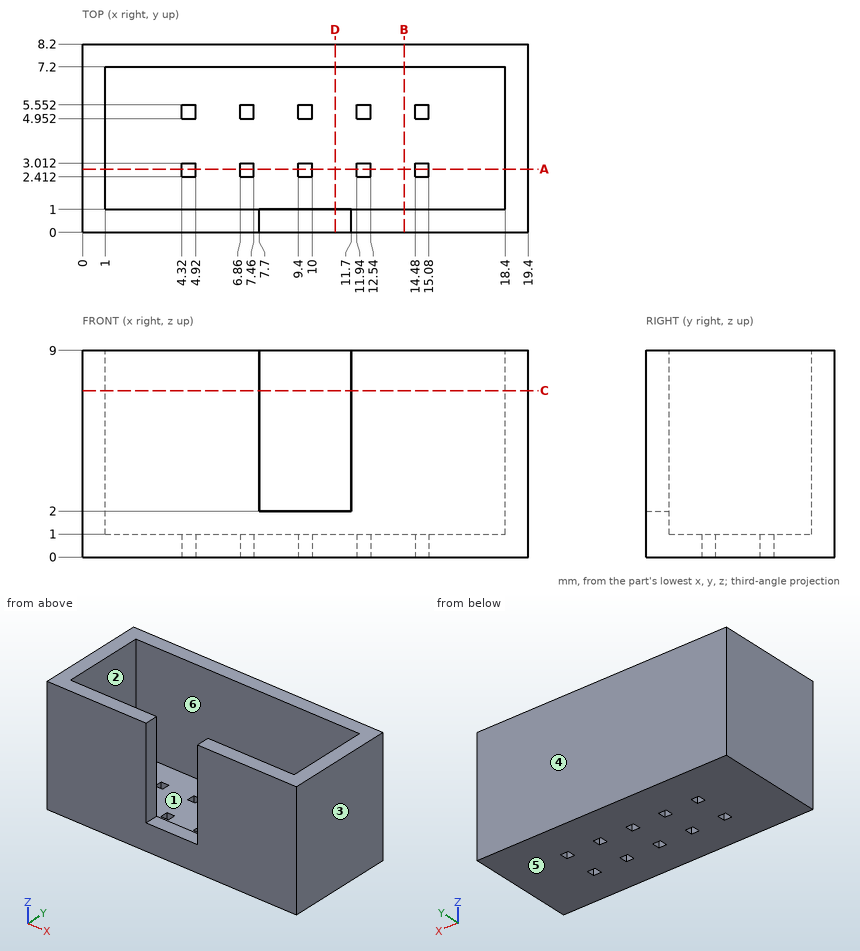
Could you check a few things on this drawing? It's one solid part, dimensions in mm from its lowest x, y, z. A direction names the side the tool comes from. Give positions to 0.01 mm unless a question says otherwise; leave off trailing zeros. Order: outer loops, then holes, each group sorted by start corner. A loop starts at its lowest first (then second) coordinate and runs counter-clockwise, first axis right, second up. Notation, with made-up numbers: (32, 77.5) - (78, 77.5) arc R27 ccw to (78, 108.5) - close; hole circle Ø2 at (-13, 27). An arc over 180 degrees is marked (long way). Answer as a JSON object with one key per item and string values. Group by question number.
Item 1: If we section it at A-A on y = 2.75: Please give me the cut outline in (x, z).
Item 2: Which directions (+Z, -Z, +X, -X, +Y, -Y) give clear straight access to the entire face, cutting with the end or side of a thin tool? Please do the marked faces 5 and 6.
Item 3: If we section it at D-D on x = 11: Please give me the cut outline in (y, z).
Item 4: If we section it at B-B on x = 14: Please give me the cut outline in (y, z).
Item 5: Please list where these lines run through material, in increasing order: probe 1 along X at (y, z) = (5.5, 3.25); probe 2 along Y at (x, z) = (13.5, 7.5); probe 3 along Y at (x, z) = (7.75, 3.5).
Item 6: If we mould it in two halves opening along X, with no side actions, what happens to the marked faces 1, 2, 3 and 4? For each: pulls with the +X half, pulls with the -X half, needs draft (parallel to the pull), parting line crosses it, or undercut.
Item 7: If we section it at C-C on z = 7.25: Please give me the cut outline in (x, y).
Result set:
{
 "1": {"outline": "(0, 0) - (4.32, 0) - (4.32, 1) - (1, 1) - (1, 9) - (0, 9) - close; (4.92, 0) - (6.86, 0) - (6.86, 1) - (4.92, 1) - close; (7.46, 0) - (9.4, 0) - (9.4, 1) - (7.46, 1) - close; (10, 0) - (11.94, 0) - (11.94, 1) - (10, 1) - close; (12.54, 0) - (14.48, 0) - (14.48, 1) - (12.54, 1) - close; (15.08, 0) - (19.4, 0) - (19.4, 9) - (18.4, 9) - (18.4, 1) - (15.08, 1) - close"},
 "2": {"face 5": "-Z, +X, -X, +Y, -Y", "face 6": "+Z"},
 "3": {"outline": "(0, 0) - (8.2, 0) - (8.2, 9) - (7.2, 9) - (7.2, 1) - (1, 1) - (1, 2) - (0, 2) - close"},
 "4": {"outline": "(0, 0) - (8.2, 0) - (8.2, 9) - (7.2, 9) - (7.2, 1) - (1, 1) - (1, 9) - (0, 9) - close"},
 "5": {"probe 1": "0 to 1, 18.4 to 19.4", "probe 2": "0 to 1, 7.2 to 8.2", "probe 3": "7.2 to 8.2"},
 "6": {"face 1": "undercut", "face 2": "undercut", "face 3": "pulls with the +X half", "face 4": "needs draft"},
 "7": {"outline": "(0, 0) - (7.7, 0) - (7.7, 1) - (1, 1) - (1, 7.2) - (18.4, 7.2) - (18.4, 1) - (11.7, 1) - (11.7, 0) - (19.4, 0) - (19.4, 8.2) - (0, 8.2) - close"}
}
